Autodesk Inventor part; units mm, degrees
ref_plane "YZ Plane" through (0, 0, 0) normal (1, 0, 0) x (0, 1, 0)
ref_plane "XZ Plane" through (0, 0, 0) normal (0, 1, 0) x (-1, 0, 0)
ref_plane "XY Plane" through (0, 0, 0) normal (0, 0, 1) x (1, 0, 0)
sketch "Sketch1" plane through (0, 0, 0) normal (0, 0, 1) x (1, 0, 0)
  circle A0 centre (0, 0) radius 2.413
  dimension "d0" = 4.826
extrude "Extrusion1" add sketch "Sketch1" along normal blind 9.525
sketch "Sketch2" plane through (0, 0, 9.525) normal (0, 0, 1) x (1, 0, 0)
  circle A0 centre (0, 0) radius 3.175
  dimension "d3" = 6.35
extrude "Extrusion2" add sketch "Sketch2" against normal blind 1.5875
sketch "Sketch3" plane through (0, 0, 9.525) normal (0, 0, 1) x (1, 0, 0)
  point P0 (0, 0)
hole "Hole1" at (0, 0, 9.525) direction (0, 0, -1) diameter 3.556 depth 3.175 tip angle 118
fillet "Fillet1" radius 0.7937 1 edges at (-2.413, 0, 0)
properties part number "button"
Here's how the part is built. I have some questions about the finished solid (model axes, mm). Coordinates: 2 decimals unless noted, no trailing zeros. Order: outer loops, then holes, each group sorted by start corner. A loop starts at its lowest first (then second) coordinate and runs counter-clockwise, first axis right, second up. Notation, with made-up numbers: M 82.5,65 L 96.5,65 A18 ccw 96.5,96 Z; hole C 31,17 d5. An arc over 180 degrees is marked long. Answer as a JSON object with one key per item and string values. Group by question number.
(1) For pin 1 (1 mm diameter, centred on x = -1, y = 2, fed in from -Z), with a flat end and sliding along its axis, tell me the tip position at first contact or that it passes through.
(2) Suppose I cut it at A-A, the plane z = 9.25. Please give me the cut outline in (x, y) (3 decimals), then the cut area to 3 significant figures.
(3) Suppose I cut it at B-B, the plane z = 2.25. Please give me the cut outline in (x, y).
(4) If we mould it in two halves opening along X, with no side actions, what happens to faces 1 (the face through (-1.915, 1.468, 4.316)), 2 (the face through (-0.19, 0.25, 5.47)), 3 (the face through (1.4, -1.4, 9.525)), 4 (the face through (1.736, 0.385, 7.915))? For each: released by +X, released by -X, zero draft, split by the parting line, or undercut.
(5) Suppose I cut it at C-C, the plane z = 6.5. Please give me the cut outline in (x, y).
(6) I need wall thicknesses on probe 1 along X at (y, z) = (0, 7.65); probe 2 along Y at (x, z) = (0, 8.3) (3 decimals). Which ranges of each line are inside material? Lowest first, please.
Values found:
{
 "1": {"pin 1": "stops at z = 0.01"},
 "2": {"outline": "C 0,0 d6.35; hole C 0,0 d3.556", "area": "21.7 mm^2"},
 "3": {"outline": "C 0,0 d4.83"},
 "4": {"face 1": "split by the parting line", "face 2": "undercut", "face 3": "zero draft", "face 4": "undercut"},
 "5": {"outline": "C 0,0 d4.83; hole C 0,0 d3.56"},
 "6": {"probe 1": "x = -2.41 to -1.78, 1.78 to 2.41", "probe 2": "y = -3.175 to -1.778, 1.778 to 3.175"}
}
